Can you work these out from the model? Positions are in its coordinate system, mm. A direction names the side the tool comes from. Give positions to 0.01 mm unless a question says otherwise; leave off trailing zeros. Loops run counter-clockwise (first coordinate to the right, second up) from the corner with the lowest first, then second, coordinate; pieces in that order, holes last. Notation, with made-up numbers: (10, 16.25) -> (16, 16.25) arc R20 ccw to (16, 38.25) -> close; hole circle Ø9 at (15, 60). An arc over 180 degrees is marked (long way). Return JSON: item names as keys, results as strings. Group by question number.
Q1. Thinking about a two-plate mould opening in X: for faces 4 (the flat face through (-25, -3, 26.255)), 5 (the flat face through (10, -3, -17)), 6 (the cylindrical face through (34.505, -6.399, 8.395)), which applies, pulls with the +X half, pulls with the -X half, needs draft (parallel to the pull), parting line crosses it, or undercut?
Q2. Suppose I cut it at B-B, the plane y = -3.25. Count the separate pieces of the cut face and the enclosed holes in it, and give its area (3 significant figures).
Q3. Will these pins go through, and if not, where does the flat tip stop? pin 1 (3.5 mm diameter, centred on x = 26.5, y = -3.5, fed in from +Z); pin 2 (3.5 mm diameter, centred on x = -25.5, y = -4, fed in from -Z); pin 3 (2 mm diameter, centred on y = -2, z = 16.5, fed in from -X).
Q4. Suppose I cut it at A-A, the plane x = 0. Please give me the cut outline in (y, z) (3 decimals).
Q5. Which directions (+Z, -Z, +X, -X, +Y, -Y) give clear straight access to the entire face, cutting with the end or side of a thin tool? Please do faces 1 (the flat face through (17.449, -3.451, -18.514)), 2 (the flat face through (35.13, -3.48, -8.34)), 3 (the flat face through (35.034, -3.479, -20.339)).
Q6. I need wall thicknesses on line 1 along Z through (x, y) = (-24.5, -3); line 2 along Z through (x, y) = (0, -4.5) (3 decimals); line 3 along X through (y, z) = (-3.75, -13.5). Which ranges of each line are inside material? Lowest first, please. Write a range as [from, to].
```python
from build123d import *

# Parameters (mm, degrees)
F0_R     = 14.5
F0_R_2   = 11.025
F1_DEPTH = 7
F2_R     = 2
F4_DEPTH = 7


# Not quite as in the source:
# - a feature names something its author has since deleted; it is built from what else it names


with BuildPart() as f1:
    # F0 (on Front) → F1 (new body)
    with BuildSketch(Plane.XZ):
        Polygon((13.8564064606, 28.5096937621), (6.9282032303, 16.5096937621), (-6.9282032303, 16.5096937621), (-13.8564064606, 28.5096937621), (-17.7619158218, 26.254846881), (-10.8337125915, 14.254846881), (-17.7619158218, 2.254846881), (-31.6183222823, 2.254846881), (-31.6183222823, -2.254846881), (-17.7619158218, -2.254846881), (-10.8337125915, -14.254846881), (-17.7619158218, -26.254846881), (-13.8564064606, -28.5096937621), (-6.9282032303, -16.5096937621), (6.9282032303, -16.5096937621), (13.8564064606, -28.5096937621), (17.7619158218, -26.254846881), (10.8337125915, -14.254846881), (17.7619158218, -2.254846881), (31.6183222823, -2.254846881), (31.6183222823, 2.254846881), (17.7619158218, 2.254846881), (10.8337125915, 14.254846881), (17.7619158218, 26.254846881), align=None)
        Circle(F0_R, mode=Mode.SUBTRACT)
        Polygon((-6.9282032303, 16.5096937621), (6.9282032303, 16.5096937621), (13.8564064606, 28.5096937621), (6.9282032303, 40.5096937621), (-6.9282032303, 40.5096937621), (-13.8564064606, 28.5096937621), align=None)
        Polygon((9.6994845224, 28.5096937621), (4.8497422612, 20.1096937621), (-4.8497422612, 20.1096937621), (-9.6994845224, 28.5096937621), (-4.8497422612, 36.9096937621), (4.8497422612, 36.9096937621), align=None, mode=Mode.SUBTRACT)
        Polygon((31.6183222823, 26.254846881), (17.7619158218, 26.254846881), (10.8337125915, 14.254846881), (17.7619158218, 2.254846881), (31.6183222823, 2.254846881), (38.5465255126, 14.254846881), align=None)
        Polygon((29.5398613133, 22.654846881), (34.3896035744, 14.254846881), (29.5398613133, 5.854846881), (19.8403767909, 5.854846881), (14.9906345297, 14.254846881), (19.8403767909, 22.654846881), align=None, mode=Mode.SUBTRACT)
        Polygon((-10.8337125915, 14.254846881), (-17.7619158218, 26.254846881), (-31.6183222823, 26.254846881), (-38.5465255126, 14.254846881), (-31.6183222823, 2.254846881), (-17.7619158218, 2.254846881), align=None)
        Polygon((-34.3896035744, 14.254846881), (-29.5398613133, 22.654846881), (-19.8403767909, 22.654846881), (-14.9906345297, 14.254846881), (-19.8403767909, 5.854846881), (-29.5398613133, 5.854846881), align=None, mode=Mode.SUBTRACT)
        Polygon((38.5465255126, -14.254846881), (31.6183222823, -2.254846881), (17.7619158218, -2.254846881), (10.8337125915, -14.254846881), (17.7619158218, -26.254846881), (31.6183222823, -26.254846881), align=None)
        Polygon((34.3896035744, -14.254846881), (29.5398613133, -22.654846881), (19.8403767909, -22.654846881), (14.9906345297, -14.254846881), (19.8403767909, -5.854846881), (29.5398613133, -5.854846881), align=None, mode=Mode.SUBTRACT)
        Polygon((-17.7619158218, -2.254846881), (-31.6183222823, -2.254846881), (-38.5465255126, -14.254846881), (-31.6183222823, -26.254846881), (-17.7619158218, -26.254846881), (-10.8337125915, -14.254846881), align=None)
        Polygon((-29.5398613133, -22.654846881), (-34.3896035744, -14.254846881), (-29.5398613133, -5.854846881), (-19.8403767909, -5.854846881), (-14.9906345297, -14.254846881), (-19.8403767909, -22.654846881), align=None, mode=Mode.SUBTRACT)
        Polygon((6.9282032303, -40.5096937621), (13.8564064606, -28.5096937621), (6.9282032303, -16.5096937621), (-6.9282032303, -16.5096937621), (-13.8564064606, -28.5096937621), (-6.9282032303, -40.5096937621), align=None)
        Polygon((4.8497422612, -36.9096937621), (-4.8497422612, -36.9096937621), (-9.6994845224, -28.5096937621), (-4.8497422612, -20.1096937621), (4.8497422612, -20.1096937621), (9.6994845224, -28.5096937621), align=None, mode=Mode.SUBTRACT)
        Circle(F0_R)
        Circle(F0_R_2, mode=Mode.SUBTRACT)
    extrude(amount=F1_DEPTH)

    # F2
    f2_edges = [f1.edges().sort_by_distance(p)[0] for p in [
        (0, -7, 40.509694),
        (10.392305, -7, 34.509694),
        (24.690119, -7, 26.254847),
        (35.082424, -7, 20.254847),
        (35.082424, -7, 8.254847),
        (35.082424, -7, -8.254847),
        (35.082424, -7, -20.254847),
        (24.690119, -7, -26.254847),
        (10.392305, -7, -34.509694),
        (0, -7, -40.509694),
        (-10.392305, -7, -34.509694),
        (-24.690119, -7, -26.254847),
        (-35.082424, -7, -20.254847),
        (-35.082424, -7, -8.254847),
        (-35.082424, -7, 8.254847),
        (-35.082424, -7, 20.254847),
        (-24.690119, -7, 26.254847),
        (-10.392305, -7, 34.509694),
        (-10.392305, 0, -34.509694),
        (10.392305, 0, -34.509694),
        (24.690119, 0, -26.254847),
        (35.082424, 0, -20.254847),
        (35.082424, 0, -8.254847),
        (35.082424, 0, 8.254847),
        (35.082424, 0, 20.254847),
        (24.690119, 0, 26.254847),
        (10.392305, 0, 34.509694),
        (-24.690119, 0, 26.254847),
        (-35.082424, 0, 20.254847),
        (-35.082424, 0, 8.254847),
        (-35.082424, 0, -8.254847),
        (-35.082424, 0, -20.254847),
        (-24.690119, 0, -26.254847),
        (0, 0, -40.509694),
        (-10.392305, 0, 34.509694),
        (0, 0, 40.509694),
        (-15.809161, -7, 27.38227),
        (15.809161, -7, 27.38227),
        (31.618322, -7, 0),
        (15.809161, -7, -27.38227),
        (-15.809161, -7, -27.38227),
        (-31.618322, -7, 0),
        (-15.809161, 0, 27.38227),
        (15.809161, 0, 27.38227),
        (31.618322, 0, 0),
        (15.809161, 0, -27.38227),
        (-15.809161, 0, -27.38227),
        (-31.618322, 0, 0),
    ]]
    fillet(f2_edges, radius=F2_R)

    # F3 (on Front) → F4 (cut)
    with BuildSketch(Plane.XZ):
        Polygon((-6.3233720139, 11.0753334069), (-6.3233720139, 19.1219889618), (-13.2919801399, 15.0986611843), align=None)
        Polygon((-19.7218142187, 4.0847936793), (-19.7218142187, -3.9618618756), (-12.7532060927, 0.0614659018), align=None)
        Polygon((-13.3984422048, -15.0371952825), (-6.4298340788, -19.0605230599), (-6.4298340788, -11.013867505), align=None)
        Polygon((6.3233720139, -19.1219889618), (13.2919801399, -15.0986611843), (6.3233720139, -11.0753334069), align=None)
        Polygon((19.7218142187, -4.0847936793), (19.7218142187, 3.9618618756), (12.7532060927, -0.0614659018), align=None)
        Polygon((13.3984422048, 15.0371952825), (6.4298340788, 19.0605230599), (6.4298340788, 11.013867505), align=None)
    extrude(amount=F4_DEPTH, mode=Mode.SUBTRACT)


solid = f1.part
```
Ans:
{
 "1": {"face 4": "needs draft", "face 5": "undercut", "face 6": "pulls with the +X half"},
 "2": {"separate pieces": "1", "enclosed holes": "13", "area": "2,280 mm^2"},
 "3": {"pin 1": "stops at z = 26.25", "pin 2": "stops at z = -26.25", "pin 3": "stops at x = -37.83"},
 "4": {"outline": "(-7, -38.51) arc R2 ccw to (-5, -40.51) -> (-2, -40.51) arc R2 ccw to (0, -38.51) -> (0, -36.91) -> (-7, -36.91) -> close; (-7, -20.11) -> (0, -20.11) -> (0, -11.025) -> (-7, -11.025) -> close; (-7, 11.025) -> (0, 11.025) -> (0, 20.11) -> (-7, 20.11) -> close; (-7, 36.91) -> (0, 36.91) -> (0, 38.51) arc R2 ccw to (-2, 40.51) -> (-5, 40.51) arc R2 ccw to (-7, 38.51) -> close"},
 "5": {"face 1": "+Y, -Y", "face 2": "+X, +Y, -Y", "face 3": "-Z, +X, +Y, -Y"},
 "6": {"line 1": "z = [-26.25, -22.65], [-5.85, 5.85], [22.65, 26.25]", "line 2": "z = [-40.51, -36.91], [-20.11, -11.025], [11.025, 20.11], [36.91, 40.51]", "line 3": "x = [-38.11, -33.95], [-15.43, -10.74], [-6.43, 6.32], [10.52, 15.43], [33.95, 38.11]"}
}
